For this review, take the finished solid that the model builds, in its own axes (mm). Face numbers are marked on the shaded views. A direction names the side the tool comes from. Round coordinates to 2 decimals unless told otherwise and drop trailing zeros. Loops run counter-clockwise (first coordinate to the right, second up) from the corner with the lowest first, then second, coordinate; pieces in that order, holes last. Notation, with made-up numbers: M 70.25,81.25 L 93.25,81.25 A13 ccw 93.25,86.25 Z; hole C 75.5,-39 d8. An arc over 180 degrees is marked long. One line per question, with ' | ' between items. Start each with the question number.
1) For probe 1 along Y at (x, z) = (0, 239.5); probe 2 along Y at (x, z) = (93.5, 104.5); probe 3 along Z at (x, y) = (-34.5, 611.5), list the stretches that pass through material, from the lowest coordinate up. Write a range as from..to.
2) We need section A-A (y = 673.1). Give the boundary of the cut face in (x, z), and give its area (3 significant figures).
3) We need section D-D (z = 119.5). Give the boundary of the cut face in (x, y), and give its area (3 significant figures).
4) For the marked faces 4 and 5, list the 3-axis set-ups (+Z, -Z, +X, -X, +Y, -Y) from which the entire face can be reached by the end or side of a thin tool; tool diameter is ignored.
5) For pin 1 Ø10 at (y, z) = (722, 188) entering from -X; pin 2 Ø12 at (x, z) = (-74.5, 191) entering from -Y; pin 3 Ø5 at (x, y) = (192, 1576.5) entering from +Z; pin 4 Ø12 at (y, z) = (983.5, 31) entering from +X, all flat-tipped, find the tip position at first contact; note any pin that passes through.
6) We need section B-B (x = 0). Give the boundary of the cut face in (y, z).
7) Mouldability with a two-part tool opening along Y and no side actions: class the marked faces 1, 2 and 3 as pulls with the +Y half, pulls with the -Y half, needs draft (parallel to the pull), parting line crosses it, or undercut.
8) We need section C-C (y = 1145.5). Give the boundary of the cut face in (x, z), and give its area (3 significant figures).
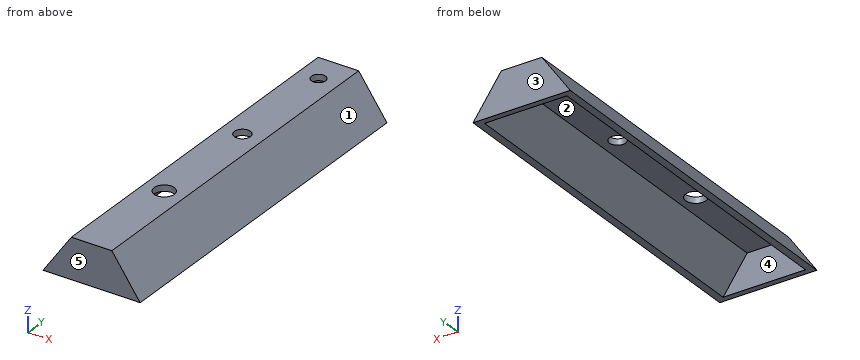
```python
from build123d import *

# Parameters (mm, degrees)
BOSS_EXTRUDE1_DEPTH     = 2286
SHELL3_T                = -38.1
CUT_EXTRUDE1_DEPTH      = 2321.175648523
CUT_EXTRUDE1_DEPTH_BACK = 2321.175648523
SKETCH2_R               = 44.45
SKETCH2_R_2             = 50.8
SKETCH2_R_3             = 63.5


with BuildPart() as part:
    # Sketch1 → Boss-Extrude1 (new body)
    with BuildSketch(Plane(origin=(0, 0, 0), x_dir=(1, 0, 0), z_dir=(0, 1, 0))):
        Polygon((-304.8, 0), (304.8, 0), (127, -254), (-127, -254), align=None)
    extrude(amount=BOSS_EXTRUDE1_DEPTH)

    # Shell3
    shell3_openings = [part.faces().sort_by_distance(p)[0] for p in [
        (0, 1143, 0),
    ]]
    offset(amount=SHELL3_T, openings=shell3_openings, kind=Kind.INTERSECTION)

    # Sketch2 → Cut-Extrude1 (cut, two sides: drawn at the far end of the back side and taken through both)
    with BuildSketch(Plane.XY.offset(254).offset(-CUT_EXTRUDE1_DEPTH_BACK)):
        with Locations(Location((0, 2101.85, 0), (0, 0, 180))):
            Circle(SKETCH2_R)
        with Locations(Location((0, 1397, 0), (0, 0, 180))):
            Circle(SKETCH2_R_2)
        with Locations(Location((0, 673.1, 0), (0, 0, 180))):
            Circle(SKETCH2_R_3)
    extrude(amount=CUT_EXTRUDE1_DEPTH + CUT_EXTRUDE1_DEPTH_BACK, mode=Mode.SUBTRACT)


solid = part.part
```
Answers below:
1) probe 1: 0..609.6, 736.6..1346.2, 1447.8..2057.4, 2146.3..2286 | probe 2: 0..38.1, 2247.9..2286 | probe 3: 215.9..254
2) outline: M -304.8,0 L -258.29,0 L -107.16,215.9 L -63.5,215.9 L -63.5,254 L -127,254 Z; M 63.5,215.9 L 107.16,215.9 L 258.29,0 L 304.8,0 L 127,254 L 63.5,254 Z | area: 25,900 mm^2
3) outline: M -221.15,0 L 221.15,0 L 221.15,2286 L -221.15,2286 Z; hole M -174.64,38.1 L 174.64,38.1 L 174.64,2247.9 L -174.64,2247.9 Z | area: 239,000 mm^2
4) face 4: -Z | face 5: +Z, -Z, +X, -X, -Y
5) pin 1: x = -176.7 | pin 2: y = 0 | pin 3: z = 164.71 | pin 4: x = 287.3
6) outline: M 0,0 L 38.1,0 L 38.1,215.9 L 609.6,215.9 L 609.6,254 L 0,254 Z; M 736.6,215.9 L 1346.2,215.9 L 1346.2,254 L 736.6,254 Z; M 1447.8,215.9 L 2057.4,215.9 L 2057.4,254 L 1447.8,254 Z; M 2146.3,215.9 L 2247.9,215.9 L 2247.9,0 L 2286,0 L 2286,254 L 2146.3,254 Z
7) face 1: needs draft | face 2: undercut | face 3: pulls with the +Y half
8) outline: M -304.8,0 L -258.29,0 L -107.16,215.9 L 107.16,215.9 L 258.29,0 L 304.8,0 L 127,254 L -127,254 Z | area: 30,800 mm^2
